Check sheet for the modelled part. Datum: model origin and axes. Units: mm. A direction names the side the tool comes from. Give positions to 0.01 mm unless a question says otherwise; leave off trailing zeros. Order: outer loops, then holes, each group sorted by start corner. A loop starts at its lowest first (then second) coordinate and runs counter-clockwise, first axis right, second up.
from build123d import *

# Parameters (mm, degrees)
EXTRUDE_1_DEPTH        = 28.5
SKETCH_2_R             = 10.5
CUT_EXTRUDE_1_DEPTH    = 87
SKETCH_3_W             = 5
SKETCH_3_H             = 1.5
EXTRUDE_2_DEPTH        = 1.5
FILLET_1_R             = 0.2
EXTRUDE_START          = -3
SKETCH_4_W             = 2
SKETCH_4_H             = 4
EXTRUDE_3_DEPTH        = 9
EXTRUDE_4_DEPTH        = 4
FILLET_2_R             = 0.2
FILLET_1_OF_MIRROR_1_R = 0.2
FILLET_2_OF_MIRROR_1_R = 0.2
FILLET_3_R             = 0.2


with BuildPart() as part:
    # 草图1 → 凸台-拉伸1 (new body)
    with BuildSketch(Plane.XY):
        Polygon((0, 0), (40, 0), (40, 12.5), (38.5, 12.5), (38.5, 1.5), (1.5, 1.5), (1.5, 12.5), (0, 12.5), align=None)
    extrude(amount=EXTRUDE_1_DEPTH)

    # 草图2 → 切除-拉伸1 (cut)
    with BuildSketch(Plane(origin=(40, 0, 0), x_dir=(0, 0, -1), z_dir=(1, 0, 0))):
        with Locations((-11.5, 12.5)):
            Circle(SKETCH_2_R)
    extrude(amount=-CUT_EXTRUDE_1_DEPTH, mode=Mode.SUBTRACT)

    # 草图3 → 凸台-拉伸2 (add)
    with BuildSketch(Plane(origin=(0, 0, 0), x_dir=(-1, 0, 0), z_dir=(0, 0, -1))):
        with Locations((-20, 0.75)):
            Rectangle(SKETCH_3_W, SKETCH_3_H)
    extrude_2 = extrude(amount=EXTRUDE_2_DEPTH)

    # 圆角1
    fillet_1_edges = [part.edges().sort_by_distance(p)[0] for p in [
        (17.5, 0, -0.75),
        (17.5, 1.5, -0.75),
        (22.5, 1.5, -0.75),
        (22.5, 0, -0.75),
    ]]
    fillet(fillet_1_edges, radius=FILLET_1_R)

    # 草图4 → 凸台-拉伸3 (add)
    with BuildSketch(Plane(origin=(0, 12.5, 0), x_dir=(1, 0, 0), z_dir=(0, 1, 0)).offset(EXTRUDE_START)):
        with Locations((37.5, -25.25)):
            Rectangle(SKETCH_4_W, SKETCH_4_H)
    extrude_3 = extrude(amount=EXTRUDE_3_DEPTH)

    # 草图5 → 凸台-拉伸4 (add)
    with BuildSketch(Plane.XY.offset(27.25)):
        Polygon((36.5, 9.5), (38.5, 6.5), (38.5, 9.5), align=None)
        Polygon((38.5, 18.5), (39.5, 17.75), (38.5, 17), align=None)
    extrude_4 = extrude(amount=-EXTRUDE_4_DEPTH)

    # 圆角2
    fillet_2_edges = [part.edges().sort_by_distance(p)[0] for p in [
        (39.5, 17.75, 25.25),
    ]]
    fillet(fillet_2_edges, radius=FILLET_2_R)

    # 镜向1: 凸台-拉伸2, 凸台-拉伸3, 凸台-拉伸4 across plane
    add(extrude_2.mirror(Plane(origin=(20, 0, 0), x_dir=(0, 0, 1), z_dir=(1, 0, 0))))
    add(extrude_3.mirror(Plane(origin=(20, 0, 0), x_dir=(0, 0, 1), z_dir=(1, 0, 0))))
    add(extrude_4.mirror(Plane(origin=(20, 0, 0), x_dir=(0, 0, 1), z_dir=(1, 0, 0))))

    # 圆角1 of 镜向1
    fillet_1_of_mirror_1_edges = [part.edges().sort_by_distance(p)[0] for p in [
        (22.5, 0, -0.75),
        (22.5, 1.5, -0.75),
        (17.5, 1.5, -0.75),
        (17.5, 0, -0.75),
    ]]
    fillet(fillet_1_of_mirror_1_edges, radius=FILLET_1_OF_MIRROR_1_R)

    # 圆角2 of 镜向1
    fillet_2_of_mirror_1_edges = [part.edges().sort_by_distance(p)[0] for p in [
        (0.5, 17.75, 25.25),
    ]]
    fillet(fillet_2_of_mirror_1_edges, radius=FILLET_2_OF_MIRROR_1_R)

    # 圆角3
    fillet_3_edges = [part.edges().sort_by_distance(p)[0] for p in [
        (36.5, 18.5, 25.25),
    ]]
    fillet(fillet_3_edges, radius=FILLET_3_R)


solid = part.part
1) Section check A-A, the plane y = 8.5. Record the cut outline in (x, z).
Recorded:
outline: (0, 0) - (1.5, 0) - (1.5, 1.79) - (0, 1.79) - close; (0, 21.21) - (1.5, 21.21) - (1.5, 23.25) - (2.83, 23.25) - (2.83, 27.25) - (1.5, 27.25) - (1.5, 28.5) - (0, 28.5) - close; (37.17, 23.25) - (38.5, 23.25) - (38.5, 21.21) - (40, 21.21) - (40, 28.5) - (38.5, 28.5) - (38.5, 27.25) - (37.17, 27.25) - close; (38.5, 0) - (40, 0) - (40, 1.79) - (38.5, 1.79) - close
2) Depth check by flat-ended pin: pin 1 Ø0.8 at (x, z) = (39, 24) entering from +Y (3 decimals); pin 2 Ø2 at (x, z) = (15, 25) entering from +Y; pin 3 Ø0.6 at (y, z) = (0.5, -1) entering from +X; pin 4 Ø3.5 at (y, z) = (9, 19) entering from +X. Enter the tip coordinate at first touch or a pass-through.
Recorded:
pin 1: stops at y = 18.425
pin 2: stops at y = 1.5
pin 3: stops at x = 22.5
pin 4: passes through
3) Set-up check for faces 1 (the face through (1, 12.5, 25)), 2 (the face through (2, 14, 27.25)), 3 (the face through (34, 1, 0)), 4 (the face through (36.5, 14, 25)): record each of +Z, -Z, +X, -X, +Y, -Y from which the full face is reachable in a straight line by a thin tool's end or side.
Recorded:
face 1: +Z, -Z, -X
face 2: +Z, +Y
face 3: -Z, +X, +Y, -Y
face 4: +Z, -Z, +Y
4) Section check C-C, the plane y = 16. Record the cut outline in (x, z).
Recorded:
outline: (1.5, 23.25) - (3.5, 23.25) - (3.5, 27.25) - (1.5, 27.25) - close; (36.5, 23.25) - (38.5, 23.25) - (38.5, 27.25) - (36.5, 27.25) - close
5) Draft check along Z on faces 5 (the face through (2, 14, 23.25)), 6 (the face through (2.5, 8, 25.3)), 7 (the face through (39.3, 2, 11.7)). Enter one of: +Z half, -Z half, draft (parallel to the pull), parting line (faces both ways), or undercut.
Recorded:
face 5: -Z half
face 6: draft
face 7: undercut
6) Section check B-B, the plane z = 24.5. Record the cut outline in (x, y), then the cut area to 3 significant figures.
Recorded:
outline: (0, 0) - (40, 0) - (40, 12.5) - (38.5, 12.5) - (38.5, 17) - (39.29, 17.59) arc R0.2 ccw to (39.29, 17.91) - (38.5, 18.5) - (36.7, 18.5) arc R0.2 ccw to (36.5, 18.3) - (36.5, 9.5) - (38.5, 6.5) - (38.5, 1.5) - (1.5, 1.5) - (1.5, 6.5) - (3.5, 9.5) - (3.5, 18.5) - (1.5, 18.5) - (0.71, 17.91) arc R0.2 ccw to (0.71, 17.59) - (1.5, 17) - (1.5, 12.5) - (0, 12.5) - close
area: 136 mm2
7) Material ranges on L1, parallel to X at y = 11, z = 24; L2, parallel to X at y = 2, z = 18; L3, parallel to Y at x = 33.5, z = 5.5, recorded low to high.
Recorded:
L1: x = 0 to 3.5, 36.5 to 40
L2: x = 0 to 1.5, 38.5 to 40
L3: y = 0 to 1.5
8) Section check D-D, the plane x = 5. Record the cut outline in (y, z).
Recorded:
outline: (0, 0) - (1.5, 0) - (1.5, 28.5) - (0, 28.5) - close
